```python
from build123d import *

# Parameters (mm, degrees)
CIRCULAR_BASE_ANGLE       = 180
CIYLINDRICAL_SUPPORT_R    = 5
CYLINDRICAL_SUPPORT_DEPTH = 50
SKETCH5_R                 = 0.6
PILOT_HOLE_DEPTH          = 5
SKETCH6_R                 = 0.895
BOTTOM_HOLE_DEPTH         = 33


with BuildPart() as part:
    # Sketch3 → Circular Base (revolve)
    with BuildSketch(Plane(origin=(0, 0, 0), x_dir=(1, 0, 0), z_dir=(0, 1, 0))):
        with BuildLine():
            Line((-7.5, 0), (7.5, 0))
            ThreePointArc((7.5, 0), (0, -7.5), (-7.5, 0))
        make_face()
    revolve(axis=Axis((-7.5, 0, 0), (-1, 0, 0)), revolution_arc=CIRCULAR_BASE_ANGLE)

    # Ciylindrical Support → Cylindrical Support (add)
    with BuildSketch(Plane(origin=(0, 0, 0), x_dir=(1, 0, 0), z_dir=(0, 1, 0))):
        with Locations(Location((0, 0, 0), (0, 0, 90))):
            Circle(CIYLINDRICAL_SUPPORT_R)
    extrude(amount=CYLINDRICAL_SUPPORT_DEPTH)

    # Sketch5 → Pilot Hole (cut)
    with BuildSketch(Plane(origin=(0, 50, 0), x_dir=(1, 0, 0), z_dir=(0, 1, 0))):
        with Locations(Location((0, 0, 0), (0, 0, 270))):
            Circle(SKETCH5_R)
    extrude(amount=-PILOT_HOLE_DEPTH, mode=Mode.SUBTRACT)

    # Sketch6 → Bottom Hole (cut)
    with BuildSketch(Plane.XZ):
        with Locations(Location((0, 0, 0), (0, 0, 270))):
            Circle(SKETCH6_R)
    extrude(amount=-BOTTOM_HOLE_DEPTH, mode=Mode.SUBTRACT)


solid = part.part
```
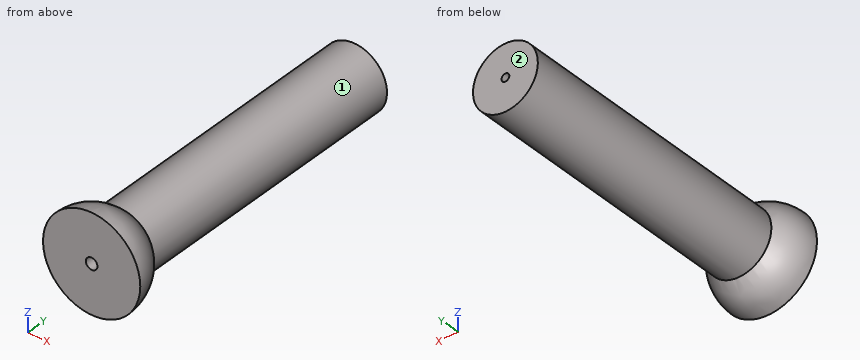
For this review, take the finished solid that the model builds, in its own axes (mm). Face numbers are marked on the shaded views. A direction names the side the tool comes from. Give positions to 0.01 mm unless a question says otherwise; leave off trailing zeros. Write each loop counter-clockwise with the first axis right and the second up, starting at its lowest first coordinate (ties: lowest second). Pieces come first, ordered by that corner, then holes.
Item 1: Take a section at C-C (y = 5). Give the boundary of the cut face in (x, z) (3 decimals).
Item 2: Take a section at D-D (y = 32). Give the boundary of the cut face in (x, z) (3 decimals), and give its area (3 significant figures).
Item 3: Machinability: for the marked faces 1 and 2, which of the approach directions +Z, -Z, +X, -X, +Y, -Y give a long, thin tool a straight path to every point of the face, cutting with its end or side? Answer none if there is none.
Item 4: Take a section at A-A (z = 0). Give the boundary of the cut face in (x, y) (3 decimals).
Item 5: Insertion check: P1, Ø2, axis at x = 5.5, z = 2.5, coming from the +Y side; P2, Ø5, axis at y = 11.5, z = -5.5, coming from the +X side; P3, Ø4, axis at x = 6, y = 31.5, coming from the +Z side. Each pin has a flat end and moves straight along its axis. Give the tip position at first contact, or say it passes through.
Item 6: Wall thickness on probe 1 along X at (y, z) = (21, 0) (3 decimals); probe 2 along X at (y, z) = (47.1, 0); probe 3 along Y at (x, z) = (5.5, 2.5): over which ranges is each line inside the solid? List them lowest first.
Item 7: Take a section at B-B (x = 0). Give the boundary of the cut face in (y, z) (3 decimals), and give its area (3 significant figures).
Established:
1. outline: circle Ø11.18 at (0, 0); hole circle Ø1.79 at (0, 0)
2. outline: circle Ø10 at (0, 0); hole circle Ø1.79 at (0, 0)
2. area: 76.0 mm2
3. face 1: +Y
3. face 2: +Z, -Z, +X, -X, +Y
4. outline: (-7.5, 0) - (-0.895, 0) - (-0.895, 33) - (0.895, 33) - (0.895, 0) - (7.5, 0) arc R7.5 ccw to (5, 5.59) - (5, 50) - (0.6, 50) - (0.6, 45) - (-0.6, 45) - (-0.6, 50) - (-5, 50) - (-5, 5.59) arc R7.5 ccw to start
5. P1: stops at y = 5.55
5. P2: stops at x = 4
5. P3: stops at z = 3
6. probe 1: x = -5 to -0.895, 0.895 to 5
6. probe 2: x = -5 to -0.6, 0.6 to 5
6. probe 3: y = 0 to 4.44
7. outline: (0, -7.5) arc R7.5 ccw to (5.59, -5) - (50, -5) - (50, -0.6) - (45, -0.6) - (45, 0.6) - (50, 0.6) - (50, 5) - (5.59, 5) arc R7.5 ccw to (0, 7.5) - (0, 0.895) - (33, 0.895) - (33, -0.895) - (0, -0.895) - close
7. area: 454 mm2
